Autodesk Inventor part; units mm, degrees
ref_plane "YZ Plane" through (0, 0, 0) normal (1, 0, 0) x (0, 1, 0)
ref_plane "XZ Plane" through (0, 0, 0) normal (0, 1, 0) x (-1, 0, 0)
ref_plane "XY Plane" through (0, 0, 0) normal (0, 0, 1) x (1, 0, 0)
sketch "スケッチ1" plane through (0, 0, 0) normal (0, 0, 1) x (1, 0, 0)
  line L0 (-22, 20) -> (22, 20)
  line L1 (22, 20) -> (22, -20)
  line L2 (22, -20) -> (-22, -20)
  line L3 (-22, -20) -> (-22, 20)
  line L4 (-22, 20) -> (22, -20) construction
  line L5 (22, 20) -> (-22, -20) construction
  point P0 (0, 0)
  point P1 (0, 0)
  dimension "d0" = 44
  dimension "d1" = 40
extrude "プレート1" add sketch "スケッチ1" along normal blind 1.5
sketch "スケッチ2" plane through (20.5, -20, 1.5) normal (1, 0, 0) x (0, 1, 0)
  line L0 (40, 0) -> (0, 0)
  line L1 (0, 0) -> (0, -25)
  line L2 (0, -25) -> (40, -25)
  line L3 (40, -25) -> (40, 0)
edge flange "フランジ1" height 25 angle 90 thickness 1.5 bend radius 1.5 thickness toward (1, 0, 0) relief tear relief width 1.5 relief depth 0.75 corner gap 1.5 corner form 0 edges at (22, 0, 0) (-22, 0, 0) wall of the first edge with corners at (20.5, 20, 1.5) (20.5, -20, 1.5) (20.5, -20, -23.5) (20.5, 20, -23.5)
bend "曲げ1"
corner "コーナー1"
equation "\"BendRadius\" = Thickness"
equation "\"BendReliefWidth\" = Thickness"
equation "\"BendReliefDepth\" = 0.5 * Thickness"
equation "\"CornerReliefSize\" = 4 * Thickness"
equation "\"MinimumRemnant\" = 2 * Thickness"
equation "\"TransitionRadius\" = BendRadius"
equation "\"JacobiRadiusSize\" = BendRadius"
equation "\"GapSize\" = Thickness"
properties part number "chest_cover_board_top"
The listing builds one solid part. Answer for the finished solid, in the listing's coordinates (mm). A direction names the side the tool comes from. Give positions to 0.01 mm unless a question says otherwise; leave off trailing zeros. Order: outer loops, then holes, each group sorted by start corner. A loop starts at its lowest first (then second) coordinate and runs counter-clockwise, first axis right, second up. Notation, with made-up numbers: (-31, 55) - (0, 55) arc R35 ccw to (0, 92) - close; hole circle Ø1 at (53.5, -37.75). An arc over 180 degrees is marked (long way). Answer as CSV lines item,"result".
Q1. A cutting plane is placed at B-B, the plane y = 11. Determine the outline of the cut face in (x, z), and give its area (3 significant figures).
Answer key:
outline,"(-22, -23.5) - (-20.5, -23.5) - (-20.5, -1.5) arc R1.5 cw to (-19, 0) - (19, 0) arc R1.5 cw to (20.5, -1.5) - (20.5, -23.5) - (22, -23.5) - (22, -1.5) arc R3 ccw to (19, 1.5) - (-19, 1.5) arc R3 ccw to (-22, -1.5) - close"
area,"134 mm^2"
Q2. A cutting plane is placed at A-A, the plane z = -15.25. Determine the outline of the cut face in (x, y), and give its area (3 significant figures).
Answer key:
outline,"(-22, -20) - (-20.5, -20) - (-20.5, 20) - (-22, 20) - close; (20.5, -20) - (22, -20) - (22, 20) - (20.5, 20) - close"
area,"120 mm^2"
Q3. Determine the mould class of faces 3 (the face through (0, 0, 0)), 4 (the face through (2, -20, 1)), 5 (the face through (0, 0, 1.5)) for opening direction Z: pulls with the +Z half, pulls with the -Z half, needs draft (parallel to the pull), parting line crosses it, or undercut.
Answer key:
face 3,"pulls with the -Z half"
face 4,"needs draft"
face 5,"pulls with the +Z half"
Q4. A cutting plane is placed at C-C, the plane x = 16. Determine the outline of the cut face in (y, z).
Answer key:
outline,"(-20, 0) - (20, 0) - (20, 1.5) - (-20, 1.5) - close"
Q5. Straight lines are drawn through the part: L1, parallel to X at y = -10, z = -8.75; L2, parallel to Z at x = 14.5, y = -6; L3, parallel to X at y = 16.5, z = -0.25. For each, find the intervals that lie inside material, in ascending order.
Answer key:
L1,"x = -22 to -20.5, 20.5 to 22"
L2,"z = 0 to 1.5"
L3,"x = -21.73 to -19.83, 19.83 to 21.73"
Q6. Which of the six approach directions +Z, -Z, +X, -X, +Y, -Y give full straight-line access (tool end or side, diameter ignored) to faces 1 (the face through (-21, 0, -23.5)), 2 (the face through (-20.07, 0.28, -0.45))?
Answer key:
face 1,"-Z, +X, -X, +Y, -Y"
face 2,"-Z, +Y, -Y"
Q7. Each of these flat-tipped pins is pushed along its axis until it touches: pin 1 Ø8 at (x, z) = (7, -3.5) entering from +Y; pin 2 Ø8 at (x, y) = (2, -15.5) entering from -Z. Where does it stop, or does it pass through?
Answer key:
pin 1,"stops at y = 20"
pin 2,"stops at z = 0"
